Source: CAD feature listing. Evaluate the final solid. Frame: model axes, mm. Give positions to 0.01 mm unless a question says otherwise; leave off trailing zeros. Write each loop counter-clockwise with the first axis right and the second up, starting at its lowest first coordinate (ties: lowest second). Pieces come first, ordered by that corner, then holes.
Autodesk Inventor part; units mm, degrees
ref_plane "YZ Plane" through (0, 0, 0) normal (1, 0, 0) x (0, 1, 0)
ref_plane "XZ Plane" through (0, 0, 0) normal (0, 1, 0) x (-1, 0, 0)
ref_plane "XY Plane" through (0, 0, 0) normal (0, 0, 1) x (1, 0, 0)
sketch "Skizze1" plane through (0, 0, 0) normal (0, 0, 1) x (1, 0, 0)
  line L0 (0, 0) -> (2, 0)
  line L1 (2, 0) -> (3.4142, 1.4142)
  line L2 (3.4142, 1.4142) -> (12.7142, 1.4142)
  line L3 (12.7142, 1.4142) -> (12.7142, 2.0642)
  line L4 (12.7142, 2.0642) -> (3.1238, 2.0642)
  line L5 (3.1238, 2.0642) -> (1.7095, 0.65)
  line L6 (1.7095, 0.65) -> (0, 0.65)
  line L7 (0, 0.65) -> (0, 0)
  dimension "d0" = 2
  dimension "d1" = 2
  dimension "d2" = 9.3
  dimension "d3" = 0.65
  dimension "d4" = 0.65
  dimension "d5" = 135
  dimension "d6" = 0.665
extrude "Extrusion1" add sketch "Skizze1" along normal blind 0.65
fillet "Rundung1" radius 0.2 4 edges at (2, 0, 0.325) (1.7095, 0.65, 0.325) (3.1238, 2.0642, 0.325) (3.4142, 1.4142, 0.325)
equation "\"Biegeradius\" = Stärke"
equation "\"BreiteBiegungsfreistellung\" = Stärke"
equation "\"TiefeBiegungsfreistellung\" = 0.5 * Stärke"
equation "\"GrößeEckenfreistellung\" = 4 * Stärke"
equation "\"MinimalRest\" = 2 * Stärke"
equation "\"Übergangsradius\" = Biegeradius"
equation "\"JacobiRadiusGröße\" = Biegeradius"
equation "\"Abstandsgröße\" = Stärke"
properties part number "Pin"
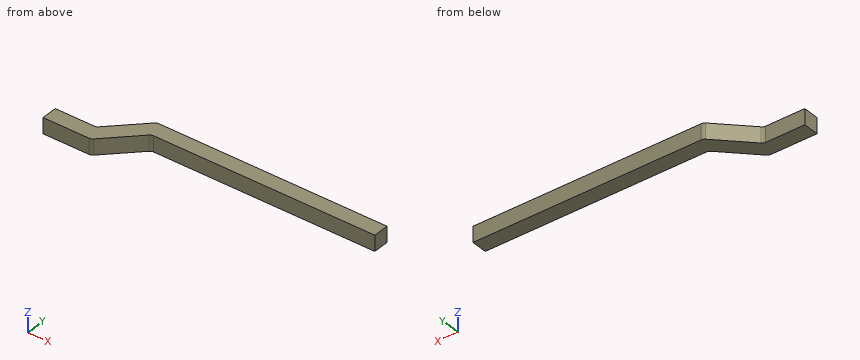
1. Line query: probe 1 along Y at (x, z) = (10.5, 0.45); probe 2 along Y at (x, z) = (1.5, 0.1); probe 3 along X at (y, z) = (1.6, 0.5). Output: solid intervals per line, ascending.
2. Section query A-A (z = 0.5). Return loops of the section in (x, y).
3. Section query C-C (y = 0.45). Return loops of the section in (x, z).
4. Section query B-B (x = 9). Return loops of the section in (y, z), plus the area to 4 significant figures.
The answers:
1. probe 1: y = 1.41 to 2.06
1. probe 2: y = 0 to 0.65
1. probe 3: x = 2.66 to 12.71
2. outline: (0, 0) - (1.92, 0) arc R0.2 ccw to (2.06, 0.06) - (3.36, 1.36) arc R0.2 cw to (3.5, 1.41) - (12.71, 1.41) - (12.71, 2.06) - (3.21, 2.06) arc R0.2 ccw to (3.07, 2.01) - (1.77, 0.71) arc R0.2 cw to (1.63, 0.65) - (0, 0.65) - close
3. outline: (0, 0) - (2.45, 0) - (2.45, 0.65) - (0, 0.65) - close
4. outline: (1.41, 0) - (2.06, 0) - (2.06, 0.65) - (1.41, 0.65) - close
4. area: 0.4225 mm2
